from build123d import *

# Parameters (mm, degrees)
SKETCH_W        = 100
SKETCH_H        = 25
PAD_DEPTH       = 8.6
SKETCH001_W     = 111.182612
SKETCH001_H     = 13.535424
POCKET_DEPTH    = 1.6
SKETCH002_R     = 2.75
POCKET001_DEPTH = 8.601
POCKET002_DEPTH = 4.5
SKETCH004_R     = 1.6
POCKET003_DEPTH = 8.601
POCKET004_DEPTH = 5
CHAMFER_SIZE    = 1


with BuildPart() as part:
    # Sketch → Pad (new body)
    with BuildSketch(Plane.XY):
        with Locations((50, 12.5)):
            Rectangle(SKETCH_W, SKETCH_H)
    extrude(amount=PAD_DEPTH)

    # Sketch001 → Pocket (cut)
    with BuildSketch(Plane.XY.offset(8.6)):
        with Locations((49.408694, 3.232288)):
            Rectangle(SKETCH001_W, SKETCH001_H)
    extrude(amount=-POCKET_DEPTH, mode=Mode.SUBTRACT)

    # Sketch002 → Pocket001 (cut, through all)
    with BuildSketch(Plane.XY.offset(8.6)):
        with Locations((50, 15)):
            Circle(SKETCH002_R)
    extrude(amount=-POCKET001_DEPTH, mode=Mode.SUBTRACT)

    # Sketch003 → Pocket002 (cut)
    with BuildSketch(Plane(origin=(0, 0, 0), x_dir=(1, 0, 0), z_dir=(0, 0, -1))):
        with BuildLine():
            ThreePointArc((60.696878, -29.303122), (64.303122, -29.303122), (64.303122, -25.696878))
            Line((64.303122, -25.696878), (34.303122, 4.303122))
            ThreePointArc((34.303122, 4.303122), (30.696878, 4.303122), (30.696878, 0.696878))
            Line((60.696878, -29.303122), (30.696878, 0.696878))
        make_face()
    extrude(amount=-POCKET002_DEPTH, mode=Mode.SUBTRACT)

    # Sketch004 → Pocket003 (cut, through all)
    with BuildSketch(Plane.XY.offset(8.6)):
        with Locations((22.5, 11.9)):
            Circle(SKETCH004_R)
        with Locations((77.5, 11.9)):
            Circle(SKETCH004_R)
    extrude(amount=-POCKET003_DEPTH, mode=Mode.SUBTRACT)

    # Sketch005 → Pocket004 (cut)
    with BuildSketch(Plane(origin=(0, 0, 0), x_dir=(1, 0, 0), z_dir=(0, 0, -1))):
        Polygon((25.514905, -10.732231), (22.996135, -8.705132), (19.98123, -9.8729), (19.485095, -13.067769), (22.003865, -15.094868), (25.01877, -13.9271), align=None)
        Polygon((80.171675, -13.769283), (80.471515, -10.550055), (77.833501, -8.680772), (74.895648, -10.030717), (74.595808, -13.249945), (77.233822, -15.119228), align=None)
    extrude(amount=-POCKET004_DEPTH, mode=Mode.SUBTRACT)

    # Chamfer
    chamfer_edges = [part.edges().sort_by_distance(p)[0] for p in [
        (15.696878, 0, 0),
        (0, 12.5, 0),
        (28.196878, 25, 0),
        (81.803122, 25, 0),
        (69.303122, 0, 0),
        (100, 12.5, 0),
        (100, 25, 4.3),
        (50, 25, 8.6),
        (100, 17.5, 8.6),
        (100, 0, 3.5),
        (0, 0, 3.5),
        (0, 17.5, 8.6),
        (0, 25, 4.3),
    ]]
    chamfer(chamfer_edges, length=CHAMFER_SIZE)


solid = part.part
Part model, mm, in its own coordinate system. A direction names the side the tool comes from. Coordinates: 2 decimals unless noted, no trailing zeros. Loops run counter-clockwise (first coordinate to the right, second up) from the corner with the lowest first, then second, coordinate; pieces in that order, holes last. Notation, with made-up numbers: (70.5, 37.25) -> (82.5, 37.25) arc R27 cw to (82.5, 74.25) -> close; hole circle Ø7 at (28, 26). An arc over 180 degrees is marked (long way). Use a Markdown table: item, result. Add a question column.
Item 1: Which spindle directions (+Z, -Z, +X, -X, +Y, -Y) get a long thin tool onto all of the face, cutting with end or side? Do faces 1 (the flat face through (49, 10, 8)), 2 (the flat face through (49, 25, 4)), 3 (the flat face through (20.73, 14.07, 2.46)). Say none if no direction does.
Item 2: Band-saw the part on A-A on z = 2.75. Write the cut outline in (x, y).
Item 3: Band-saw the part on D-D on x = 50. Write the cut outline in (y, z), plus the area to 3 significant figures.
Item 4: Flat gauge pins, fed straight in: P1, Ø1.3, axis at x = 29.5, z = 8, coming from the -Y side; P2, Ø4, axis at x = 78, y = 4.5, coming from the +Z side; P3, Ø5, axis at x = 22.5, y = 11.9, coming from the -Z side. Where does each tip first touch, or does it go through?
Item 5: Probe probe 1 along Y at (x, z) = (22.5, 6.05); probe 2 along Z at (x, y) = (87, 2.5); probe 3 along Z at (x, y) = (43, 7). List the from-to ranges inside material, lowest first.
Item 6: Band-saw the part on B-B on x = 16.5. Write the cut outline in (y, z).
Item 7: Band-saw the part on C-C on y = 7.25. Write the cut outline in (x, z).
Item 8: Pull direction X, two halves, no side cores. Call faces 4 (the flat face through (49, 19, 8.6)), 5 (the flat face through (78, 10, 5)): +X half, -X half, draft (parallel to the pull), parting line (faces both ways), or undercut.
Geometry says:
| question | item | result |
|---|---|---|
| 1 | face 1 | +Z, +X, -X, -Y |
| 1 | face 2 | +Z, -Z, +X, -X, +Y |
| 1 | face 3 | -Z |
| 2 | outline | (0, 1) -> (1, 0) -> (31.39, 0) -> (47.47, 16.08) arc R2.75 cw to (48.92, 17.53) -> (56.39, 25) -> (1, 25) -> (0, 24) -> close; (38.61, 0) -> (99, 0) -> (100, 1) -> (100, 24) -> (99, 25) -> (63.61, 25) -> (52.53, 13.92) arc R2.75 cw to (51.08, 12.47) -> close; hole (19.49, 13.07) -> (19.98, 9.87) -> (23, 8.71) -> (25.51, 10.73) -> (25.02, 13.93) -> (22, 15.09) -> close; hole (74.6, 13.25) -> (74.9, 10.03) -> (77.83, 8.68) -> (80.47, 10.55) -> (80.17, 13.77) -> (77.23, 15.12) -> close |
| 3 | outline | (0, 1) -> (1, 0) -> (11.39, 0) -> (11.39, 4.5) -> (12.25, 4.5) -> (12.25, 8.6) -> (10, 8.6) -> (10, 7) -> (0, 7) -> close; (17.75, 4.5) -> (18.61, 4.5) -> (18.61, 0) -> (24, 0) -> (25, 1) -> (25, 7.6) -> (24, 8.6) -> (17.75, 8.6) -> close |
| 3 | area | 142 mm² |
| 4 | P1 | y = 10 |
| 4 | P2 | z = 7 |
| 4 | P3 | z = 5 |
| 5 | probe 1 | 0 to 10.3, 13.5 to 25 |
| 5 | probe 2 | 0 to 7 |
| 5 | probe 3 | 4.5 to 7 |
| 6 | outline | (0, 1) -> (1, 0) -> (24, 0) -> (25, 1) -> (25, 7.6) -> (24, 8.6) -> (10, 8.6) -> (10, 7) -> (0, 7) -> close |
| 7 | outline | (0, 1) -> (1, 0) -> (38.64, 0) -> (38.64, 4.5) -> (45.86, 4.5) -> (45.86, 0) -> (99, 0) -> (100, 1) -> (100, 7) -> (0, 7) -> close |
| 8 | face 4 | draft |
| 8 | face 5 | undercut |
